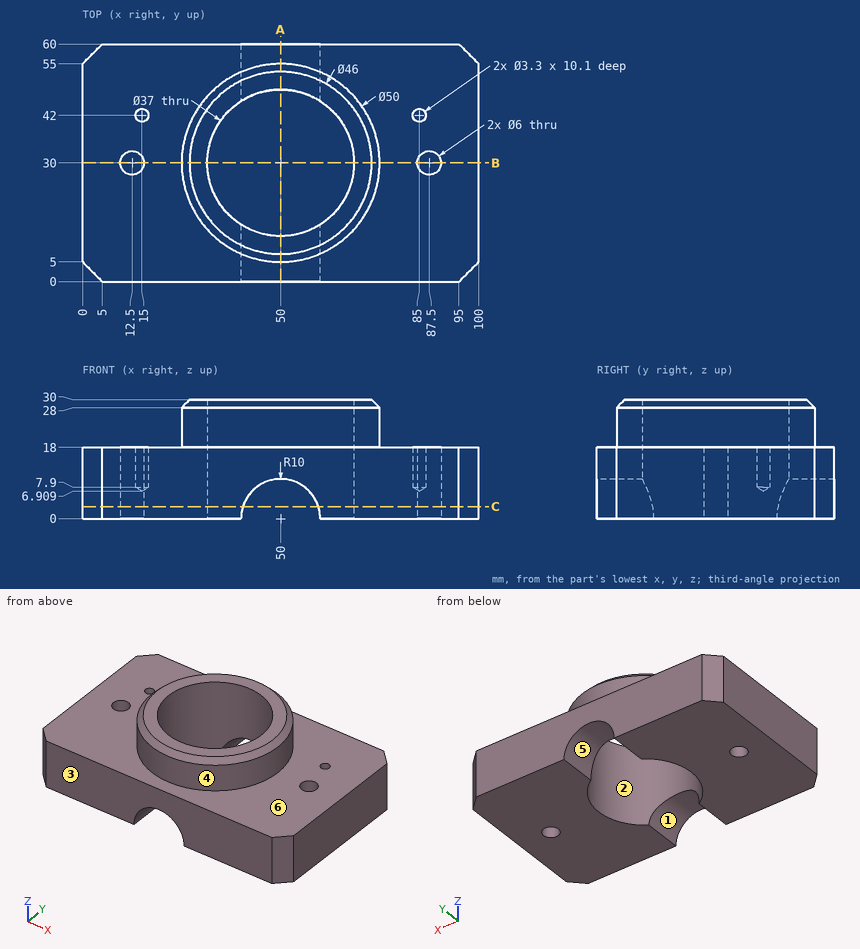
The figure shows three views and two pictorial views of one solid part (mm, origin at its lowest corner). Answer the questions. A direction names the side the tool comes from. Round coordinates to 2 decimals unless told otherwise and drop trailing zeros. Loops run counter-clockwise (first coordinate to the right, second up) from the corner with the lowest first, then second, coordinate; pieces in that order, holes last. Notation, with made-up numbers: (15, 70.5) - (49, 70.5) arc R18 ccw to (49, 99.5) - close; hole circle Ø10 at (60.25, -11.5). An arc over 180 degrees is marked (long way). One line per question, with ' | ' between items. Start each with the question number.
Q1. Find the intervals of material crossed by L1, parallel to Y at x = 87.5, z = 4.25; L2, parallel to X at y = 32, z = 12 (1 decimal); L3, parallel to Y at x = 50, z = 21.5, in increasing order.
Q2. For the marked faces 5 and 6, determine the directions among +Z, -Z, +X, -X, +Y, -Y from which every point of the face is accessible in a straight line to the end or side of a thin tool.
Q3. Section B-B on y = 30 is taken. Give the vertices of the cut face in (x, z).
Q4. Section C-C on z = 3 is taken. Give the vertices of the cut face in (x, y), plus the area to 3 significant figures.
Q5. Flat-ended cylindrical pins translate along their axes: pin 1 (12 mm diameter, centred on x = 48.5, z = 6, fed in from +Y); pin 2 (4 mm diameter, centred on x = 85, y = 42, fed in from +Z); pin 3 (12 mm diameter, centred on x = 47, y = 51, fed in from -Z). Find the tip coordinate at first contact, or state that the pin passes through.
Q6. For a pull along Y with two mould halves and no side action, classify the marked faces 1, 2, 3 and 4 as +Y half, -Y half, draft (parallel to the pull), parting line (faces both ways), or undercut.
Q7. Section A-A on x = 50 is taken. Give the vertices of the cut face in (y, z), plus the area to 3 significant figures.
Established:
1) L1: 0 to 27, 33 to 60 | L2: 0 to 10.3, 14.7 to 31.6, 68.4 to 85.3, 89.7 to 100 | L3: 5 to 11.5, 48.5 to 55
2) face 5: -Z, +Y, -Y | face 6: +Z
3) outline: (0, 0) - (9.5, 0) - (9.5, 18) - (0, 18) - close; (15.5, 0) - (31.5, 0) - (31.5, 30) - (27, 30) - (25, 28) - (25, 18) - (15.5, 18) - close; (68.5, 0) - (84.5, 0) - (84.5, 18) - (75, 18) - (75, 28) - (73, 30) - (68.5, 30) - close; (90.5, 0) - (100, 0) - (100, 18) - (90.5, 18) - close
4) outline: (0, 5) - (5, 0) - (40.46, 0) - (40.46, 14.15) arc R18.5 cw to (40.46, 45.85) - (40.46, 60) - (5, 60) - (0, 55) - close; (59.54, 0) - (95, 0) - (100, 5) - (100, 55) - (95, 60) - (59.54, 60) - (59.54, 45.85) arc R18.5 cw to (59.54, 14.15) - close; hole circle Ø6 at (12.5, 30); hole circle Ø6 at (87.5, 30) | area: 4,350 mm²
5) pin 1: y = 60 | pin 2: z = 18 | pin 3: z = 4.36
6) face 1: draft | face 2: undercut | face 3: -Y half | face 4: parting line
7) outline: (0, 10) - (11.5, 10) - (11.5, 30) - (7, 30) - (5, 28) - (5, 18) - (0, 18) - close; (48.5, 10) - (60, 10) - (60, 18) - (55, 18) - (55, 28) - (53, 30) - (48.5, 30) - close | area: 336 mm²
